Model file for the job. Use its own axes, mm. Give positions to 0.01 mm unless a question says otherwise; leave off trailing zeros. Loops run counter-clockwise (first coordinate to the right, second up) from the corner with the lowest first, then second, coordinate; pieces in that order, holes last. Notation, with made-up numbers: (-8, 66) - (30, 66) arc R18 ccw to (30, 86) - close; hole circle Ø7 at (54, -7). An arc over 180 degrees is marked (long way). Use a Markdown table: item, result.
from build123d import *

# Parameters (mm, degrees)
F1_DEPTH = 3


with BuildPart() as f1:
    # F0 (on Front) → F1 (new body, symmetric)
    with BuildSketch(Plane.XZ):
        with BuildLine():
            Line((0, 40), (0, 0))
            Line((0, 0), (106, 0))
            Line((106, 0), (106, 40))
            Line((106, 40), (101, 40))
            ThreePointArc((101, 40), (53, 16), (5, 40))
            Line((5, 40), (0, 40))
        make_face()
    extrude(amount=F1_DEPTH, both=True)


solid = f1.part
(1) Slice it at C-C, the plane z = 34.5. Write the cut outline in (x, y).
Computed:
| item | result |
|---|---|
| outline | (0, -3) - (9.67, -3) - (9.67, 3) - (0, 3) - close; (96.33, -3) - (106, -3) - (106, 3) - (96.33, 3) - close |
(2) Slice it at D-D, the plane x = 51. Write the cut outline in (y, z), plus the area to 3 significant figures.
Computed:
| item | result |
|---|---|
| outline | (-3, 0) - (3, 0) - (3, 16.03) - (-3, 16.03) - close |
| area | 96.2 mm² |
(3) Slice it at A-A, the plane z = 20.5. Write the cut outline in (x, y).
Computed:
| item | result |
|---|---|
| outline | (0, -3) - (30.2, -3) - (30.2, 3) - (0, 3) - close; (75.8, -3) - (106, -3) - (106, 3) - (75.8, 3) - close |
(4) Slice it at B-B, the plane y = 1.25. Write the cut outline in (x, z).
Computed:
| item | result |
|---|---|
| outline | (0, 0) - (106, 0) - (106, 40) - (101, 40) arc R60 cw to (5, 40) - (0, 40) - close |
(5) Mould opens along X. For faces 1 (the cylindrical face through (53.779, -0.042, 16.005)), 2 (the flat face through (106, 0, 20)), 3 (the flat face through (0, 0, 20)) say: pulls with the +X half, pulls with the -X half, needs draft (parallel to the pull), parting line crosses it, or undercut.
Computed:
| item | result |
|---|---|
| face 1 | undercut |
| face 2 | pulls with the +X half |
| face 3 | pulls with the -X half |
(6) Drill centre lines: probe 1 along X at (y, z) = (-0.95, 31.5); probe 2 along X at (y, z) = (-1.3, 29.5); probe 3 along Z at (x, y) = (97, -0.65). Where is each one in solid material? Low to high. Write a range as [from, to].
Computed:
| item | result |
|---|---|
| probe 1 | [0, 12.75], [93.25, 106] |
| probe 2 | [0, 15.08], [90.92, 106] |
| probe 3 | [0, 35.21] |
